The drawing under review shows one solid part. Ordinate dimensions are in mm from its lowest x, y, z. Give positions to 0.01 mm unless a question says otherwise; leave off trailing zeros. Write each loop counter-clockwise with the first axis right and the second up, starting at its lowest first coordinate (ties: lowest second). Pieces come first, ordered by that corner, then holes. Notation, with made-up numbers: (88.25, -37) -> (130.25, -37) arc R25 ccw to (130.25, -16) -> close; hole circle Ø11 at (-35, 22.5). An arc over 180 degrees is marked (long way). Answer as a JSON object with one key per item and string values.
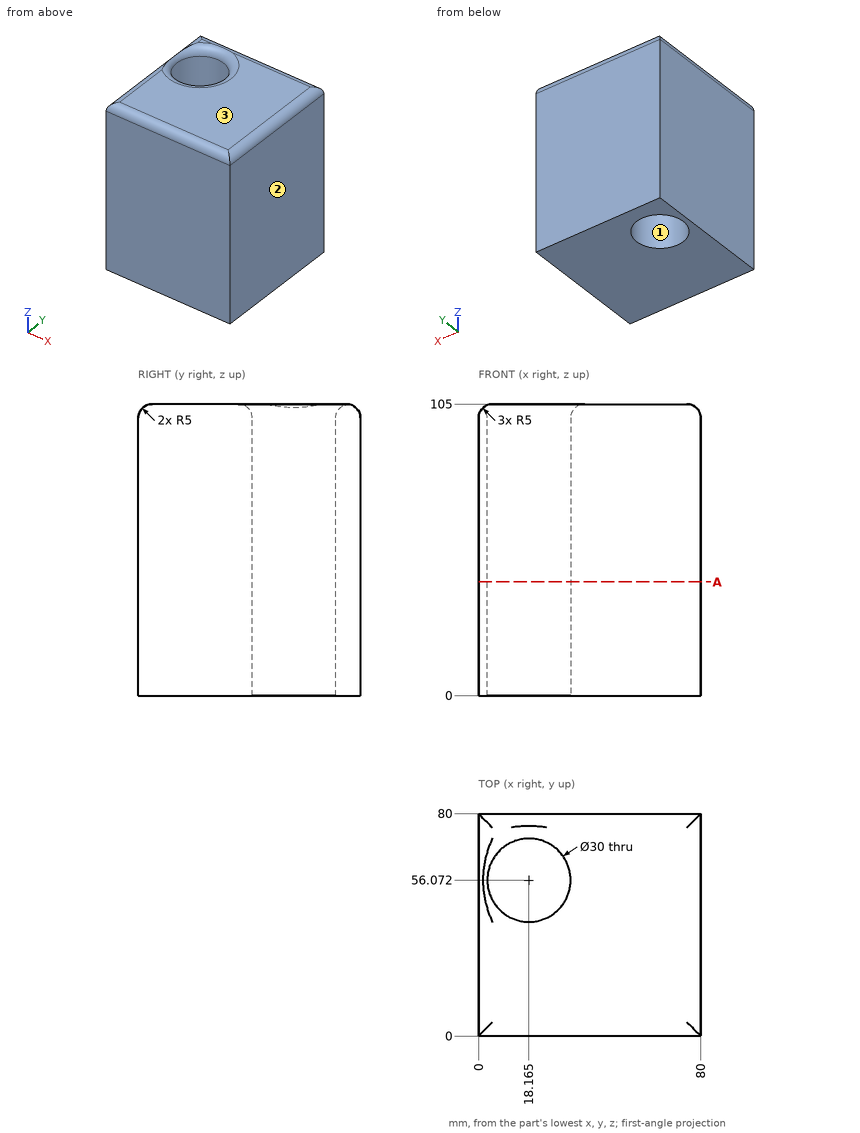
(1) For line 1 along Y through (x, z) = (26, 66.5); line 2 along Y through (x, z) = (16.5, 11) (1 decimal); line 3 along X through (y, z) = (53.5, 6), list the stretches that pass through material, from the lowest coordinate up.
Here are the results:
{"line 1": "y = 0 to 43.28, 68.86 to 80", "line 2": "y = 0 to 41.2, 71 to 80", "line 3": "x = 0 to 3.39, 32.94 to 80"}
(2) The part is to be moulded in two halves that separate along X. For the marked faces 1, 2 and 3, say which applies: +X half, -X half, draft (parallel to the pull), parting line (faces both ways), or undercut.
Here are the results:
{"face 1": "undercut", "face 2": "+X half", "face 3": "draft"}
(3) We need section A-A, the plane z = 41. State the section outline as (x, y) points (1 decimal), then the cut area to 3 significant figures.
Here are the results:
{"outline": "(0, 0) -> (80, 0) -> (80, 80) -> (0, 80) -> close; hole circle Ø30 at (18.2, 56.1)", "area": "5,690 mm²"}
(4) Clearance check with a flat-ended pin moving along its axis: pin 1 (1 mm diameter, centred on x = 15.5, y = 22.5, fed in from -Z). State where the tip first meets the part, or that it passes through.
Here are the results:
{"pin 1": "stops at z = 0"}
